The drawing under review shows one solid part. Ordinate dimensions are in mm from its lowest x, y, z. A direction names the side the tool comes from. Round coordinates to 2 decimals unless told otherwise and drop trailing zeros. Order: outer loops, then holes, each group sorted by start corner. A loop starts at its lowest first (then second) coordinate and runs counter-clockwise, first axis right, second up. Notation, with made-up numbers: M 20.5,-10.5 L 54.5,-10.5 A26 ccw 54.5,23.5 Z; hole C 67.25,67.25 d8. An arc over 180 degrees is marked long. Answer as a JSON object with one key per item and string values. Group by question number.
1) Consider section C-C, the plane z = 42. Write out the cut boundary in (x, y), then the cut area to 3 significant figures.
2) For the marked faces 1, 2 and 3, list the 3-axis set-ups (+Z, -Z, +X, -X, +Y, -Y) from which the entire face can be reached by the end or side of a thin tool; tool diameter is ignored.
3) Insertion check: pin 1 Ø20.5 at (x, y) = (62.5, 13) entering from +Z; pin 2 Ø12 at (x, z) = (61.5, 43) entering from +Y; pin 3 Ø7.5 at (y, z) = (15.5, 35.5) entering from +X; pin 4 Ø5 at (x, y) = (44, 54) entering from -Z. Each pin has a flat end and moves straight along its axis. Give the tip position at first contact, or say it passes through.
4) Consider section B-B, the plane x = 133.5. Write out the cut boundary in (y, z).
5) Consider section A-A, the plane y = 34. Write out the cut boundary in (x, z).
6) To check wall thickness, follow line 1 (Y direction, x = 75, z = 34.5); line 2 (X direction, y = 5, z = 45.5); line 3 (Z direction, x = 30.5, y = 21). State the ranges of each line that lie inside material, in increasing order.
7) Consider section D-D, the plane y = 65. Write out the cut boundary in (x, z), then the cut area to 3 significant figures.
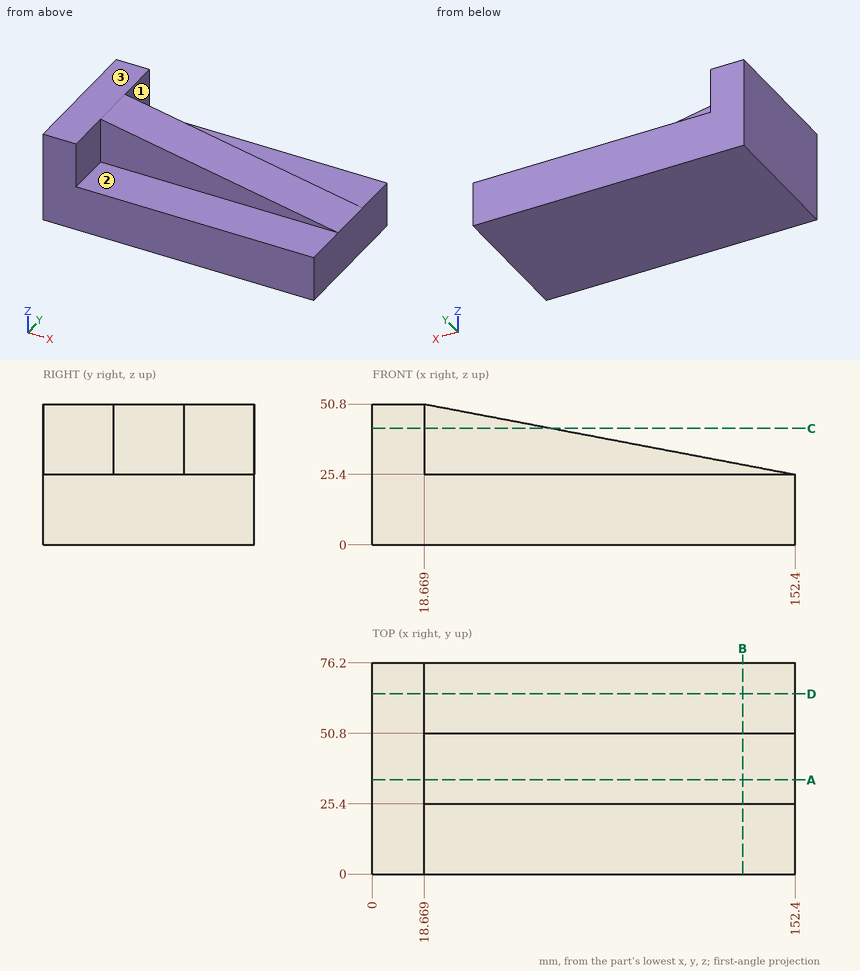
Results list:
{
 "1": {"outline": "M 0,0 L 18.67,0 L 18.67,25.4 L 65,25.4 L 65,50.8 L 18.67,50.8 L 18.67,76.2 L 0,76.2 Z", "area": "2,600 mm^2"},
 "2": {"face 1": "+Z, +X, +Y", "face 2": "+Z, +X, -Y", "face 3": "+Z, +X, -X, +Y, -Y"},
 "3": {"pin 1": "z = 25.4", "pin 2": "y = 50.8", "pin 3": "x = 18.67", "pin 4": "z = 0"},
 "4": {"outline": "M 0,0 L 76.2,0 L 76.2,25.4 L 50.8,25.4 L 50.8,28.99 L 25.4,28.99 L 25.4,25.4 L 0,25.4 Z"},
 "5": {"outline": "M 0,0 L 152.4,0 L 152.4,25.4 L 18.67,50.8 L 0,50.8 Z"},
 "6": {"line 1": "25.4 to 50.8", "line 2": "0 to 18.67", "line 3": "0 to 25.4"},
 "7": {"outline": "M 0,0 L 152.4,0 L 152.4,25.4 L 18.67,25.4 L 18.67,50.8 L 0,50.8 Z", "area": "4,350 mm^2"}
}
